The listing builds one solid part. Answer for the finished solid, in the listing's coordinates (mm). A direction names the side the tool comes from. Coordinates: 2 decimals unless noted, no trailing zeros. Write each loop counter-clockwise with the first axis right and the second up, starting at its lowest first coordinate (ties: lowest second). Pieces come first, ordered by that corner, then holes.
```python
from build123d import *

# Parameters (mm, degrees)
F0_W      = 20
F0_H      = 10
F1_DEPTH  = 5
F3_DEPTH  = 5
F4_R      = 1.27
F5_DEPTH  = 7.287
F7_DEPTH  = 25.4
F9_DEPTH  = 25.4
F10_W     = 0.6200999394
F10_H     = 0.5964474939
F11_DEPTH = 25.4
F12_W     = 0.5901486054
F12_H     = 4.5354563772
F13_DEPTH = 25.4


with BuildPart() as f1:
    # F0 (on Top) → F1 (new body)
    with BuildSketch(Plane.XY):
        with Locations((1.042785123, -6.5861073174)):
            Rectangle(F0_W, F0_H)
    extrude(amount=F1_DEPTH)

    # F2 (on face) → F3 (join)
    with BuildSketch(Plane(origin=(-8.957214877, 0, 0), x_dir=(0, -1, 0), z_dir=(-1, 0, 0))):
        Polygon((4.3001073174, 0), (6.5861073174, 0), (8.8721073174, 0), (8.8721073174, 5), (6.5861073174, 5), (4.3001073174, 5), align=None)
    extrude(amount=F3_DEPTH)

    # F4 (on face) → F5 (cut, through all)
    with BuildSketch(Plane.XZ.offset(8.8721073174)):
        with BuildLine():
            ThreePointArc((-11.457214877, 0), (-13.9450408659, 2.5), (-11.457214877, 5))
            Line((-11.457214877, 5), (-14.9464672431, 5.5829798803))
            Line((-14.9464672431, 5.5829798803), (-15.761434359, 0.3301068575))
            Line((-15.761434359, 0.3301068575), (-11.6382623091, -0.7145671407))
            Line((-11.6382623091, -0.7145671407), (-11.457214877, 0))
        make_face()
        with Locations((-11.4450110796, 2.5)):
            Circle(F4_R)
    extrude(amount=-F5_DEPTH, mode=Mode.SUBTRACT)

    # F6 (on face) → F7 (cut)
    with BuildSketch(Plane.XZ.offset(8.8721073174)):
        Polygon((-8.957214877, 5), (-11.457214877, 5), (-8.957214877, 4.4035525061), align=None)
    extrude(amount=-F7_DEPTH, mode=Mode.SUBTRACT)

    # F8 (on face) → F9 (cut)
    with BuildSketch(Plane.XZ.offset(8.8721073174)):
        Polygon((-8.957214877, 5.1671843976), (-8.957214877, 4.4035525061), (-8.957214877, 0), (-8.3371149376, 0), (-8.3371149376, 5.1671843976), align=None)
    extrude(amount=F9_DEPTH, mode=Mode.SUBTRACT)

    # F10 (on face) → F11 (cut)
    with BuildSketch(Plane.XZ.offset(8.8721073174)):
        with Locations((-8.6471649073, 4.7017762531)):
            Rectangle(F10_W, F10_H)
    extrude(amount=-F11_DEPTH, mode=Mode.SUBTRACT)

    # F12 (on face) → F13 (cut)
    with BuildSketch(Plane(origin=(0, -4.3001073174, 0), x_dir=(-1, 0, 0), z_dir=(0, 1, 0))):
        with Locations((8.6621405743, 2.1358243175)):
            Rectangle(F12_W, F12_H)
    extrude(amount=F13_DEPTH, mode=Mode.SUBTRACT)


solid = f1.part
```
(1) Section D-D, the plane y = -9.25 is taken. Write down the section's boundary in (x, z), plus the area to 3 significant figures.
(2) Each of these flat-tipped pins is pushed along its axis until it touches: pin 1 (1.4 mm diameter, centred on y = -2.5, z = 3, fed in from -X); pin 2 (1.5 mm diameter, centred on x = -12.5, z = 3.5, fed in from +Y). Where does it stop, or does it pass through?
(3) Find the intervals of material crossed by probe 1 along X at (y, z) = (-8, 1.6); probe 2 along X at (y, z) = (-8, 4.1); probe 3 along X at (y, z) = (-7, 3.1), in increasing order.
(4) Section C-C, the plane z = 1.5 is taken. Write down the section's boundary in (x, y), plus the area to 3 significant figures.
(5) For a pull along Z with two mould halves and no side action, classify faces 1 (the cylindrical face through (-10.272, -6.618, 2.014)), 2 (the flat face through (-8.337, -9.2, 2.9)), 3 (the cylindrical face through (-13.944, -6.618, 2.445)) as pulls with the +Z half, pulls with the -Z half, needs draft (parallel to the pull), parting line crosses it, or undercut.
(6) Section A-A, the plane z = 2.5 is taken. Write down the section's boundary in (x, y).
(7) Which of the six approach directions +Z, -Z, +X, -X, +Y, -Y give full straight-line access (tool end or side, diameter ignored) to faces 4 (the flat face through (-10, -8.872, 2)), 5 (the flat face through (1, -11.586, 2)), 6 (the flat face through (-8.367, -3, 2)), 7 (the flat face through (-10.2, -6.6, 4.7))?
(8) Section B-B, the plane y = -5.5 is taken. Write down the section's boundary in (x, z).
Solution:
1. outline: (-8.34, 0) - (11.04, 0) - (11.04, 5) - (-8.34, 5) - close
1. area: 96.9 mm2
2. pin 1: stops at x = -8.37
2. pin 2: stops at y = -4.3
3. probe 1: x = -13.78 to -12.34, -10.55 to 11.04
3. probe 2: x = -13.37 to 11.04
3. probe 3: x = -13.87 to -12.56, -10.33 to 11.04
4. outline: (-13.74, -8.87) - (-12.23, -8.87) - (-12.23, -4.3) - (-13.74, -4.3) - close; (-10.66, -8.87) - (-8.34, -8.87) - (-8.34, -11.59) - (11.04, -11.59) - (11.04, -1.59) - (-8.37, -1.59) - (-8.37, -4.3) - (-10.66, -4.3) - close
4. area: 211 mm2
5. face 1: undercut
5. face 2: needs draft
5. face 3: parting line crosses it
6. outline: (-13.95, -8.87) - (-12.72, -8.87) - (-12.72, -4.3) - (-13.95, -4.3) - close; (-10.18, -8.87) - (-8.34, -8.87) - (-8.34, -11.59) - (11.04, -11.59) - (11.04, -1.59) - (-8.37, -1.59) - (-8.37, -4.3) - (-10.18, -4.3) - close
7. face 4: +Z, -Z, -X, -Y
7. face 5: +Z, -Z, +X, -X, -Y
7. face 6: +Z, -Z, -X, +Y
7. face 7: +Z, +Y, -Y
8. outline: (-11.46, 0) - (11.04, 0) - (11.04, 5) - (-8.34, 5) - (-8.34, 4.4) - (-8.96, 4.4) - (-11.46, 5) arc R2.5 ccw to start; hole circle Ø2.54 at (-11.45, 2.5)
